Autodesk Inventor part; units mm, degrees
ref_plane "YZ Plane" through (0, 0, 0) normal (1, 0, 0) x (0, 1, 0)
ref_plane "XZ Plane" through (0, 0, 0) normal (0, 1, 0) x (-1, 0, 0)
ref_plane "XY Plane" through (0, 0, 0) normal (0, 0, 1) x (1, 0, 0)
sketch "Szkic1" plane through (0, 0, 0) normal (0, 0, 1) x (1, 0, 0)
  circle A0 centre (0, 0) radius 32.5
  dimension "d0" = 65
extrude "Wyciągnięcie proste1" add sketch "Szkic1" along normal blind 110
ref_plane "Płaszczyzna konstrukcyjna5" through (0, 0, 55) normal (0, 0, -1) x (-1, 0, 0)
sketch "Szkic3" plane through (0, 0, 55) normal (0, 0, -1) x (-1, 0, 0)
  line L0 (0, 0) -> (28, 0)
  line L1 (28, 0) -> (28, 16.5)
  circle A0 centre (0, 0) radius 32.5
  line L2 (28, 0) -> (28, -35.6443)
  line L3 (28, -35.6443) -> (-28, -35.6443)
  line L4 (-28, -35.6443) -> (-28, 35.8328)
  line L5 (-28, 35.8328) -> (28, 35.8328)
  line L6 (28, 35.8328) -> (28, 0)
  dimension "d3" = 28
  dimension "d4" = 56
  dimension "d5" = 56
extrude "Wyciągnięcie proste2" cut sketch "Szkic3" along normal blind 25 and the other way blind 52 contours L2 A0 L4 L1 | A0 L4 L5 L6 | L2 L3 L4 A0
sketch "Szkic5" plane through (0, 0, 0) normal (0, 0, -1) x (-1, 0, 0)
  circle A0 centre (0, 0) radius 32.5
extrude "Wyciągnięcie proste3" cut sketch "Szkic5" against normal blind 27
sketch "Szkic6" plane through (0, 0, 27) normal (0, 0, -1) x (-1, 0, 0)
  circle A0 centre (0, 0) radius 15
  circle A1 centre (0, 0) radius 16.5
  dimension "d12" = 30
  dimension "d13" = 33
extrude "Wyciągnięcie proste4" add sketch "Szkic6" along normal blind 15
sketch "Szkic7" plane through (0, 0, 27) normal (0, 0, -1) x (-1, 0, 0)
  line L0 (7, -15.9899) -> (-7, -15.9899)
  line L1 (-7, -15.9899) -> (-7, -29.9899)
  line L2 (-7, -29.9899) -> (7, -29.9899)
  line L3 (7, -29.9899) -> (7, -15.9899)
  line L4 (7, -15.9899) -> (-7, -29.9899) construction
  line L5 (-7, -15.9899) -> (7, -29.9899) construction
  point P0 (0, 0)
  point P1 (0, -22.9899)
  dimension "d16" = 14
  dimension "d17" = 14
extrude "Wyciągnięcie proste5" cut sketch "Szkic7" along normal blind 5 and the other way blind 7.5
sketch "Szkic8" plane through (28, -16.5, 107) normal (-1, 0, 0) x (0, 0, 1)
  line L0 (-77, 0) -> (-77, 33)
  line L1 (-77, 16.5) -> (-37, 16.5)
  line L2 (0, 0) -> (0, 33)
  line L3 (-37, 16.5) -> (-37, 17.5)
  line L4 (-37, 17.5) -> (-37, 15.5)
  line L5 (-37, 15.5) -> (-77, 15.5)
  line L6 (-77, 15.5) -> (-77, 18.2624)
  line L7 (-77, 15.5) -> (-77, 17.5)
  line L8 (-77, 33) -> (-77, 0)
  line L9 (-77, 17.5) -> (-37, 17.5)
  line L10 (-20, 18.2624) -> (0, 18.2624)
  line L11 (0, 18.2624) -> (0, 16.2624)
  line L12 (0, 16.2624) -> (-20, 16.2624)
  line L13 (-20, 16.2624) -> (-20, 18.2624)
  point P0 (-107, 16.5)
  dimension "d22" = 40
  dimension "d23" = 1
  dimension "d24" = 2
  dimension "d25" = 2
  dimension "d28" = 2
  dimension "d29" = 20
extrude "Wyciągnięcie proste6" add sketch "Szkic8" along normal blind 56
sketch "Szkic9" plane through (0, 0, 110) normal (0, 0, 1) x (1, 0, 0)
  line L0 (12, -27) -> (-12, -27)
  line L1 (-12, -27) -> (-12, -3)
  line L2 (-12, -3) -> (12, -3)
  line L3 (12, -3) -> (12, -27)
  line L4 (12, -27) -> (-12, -3) construction
  line L5 (-12, -27) -> (12, -3) construction
  point P0 (0, 0)
  point P1 (0, -15)
  dimension "d30" = 24
  dimension "d31" = 24
extrude "Wyciągnięcie proste7" cut sketch "Szkic9" against normal blind 56
fillet "Zaokrąglenie1" radius 1 4 edges at (12, -27, 108.5) (-12, -27, 108.5) (12, -3, 108.5) (-12, -3, 108.5)
sketch "Szkic13" plane through (28, -1, 30) normal (0, -1, 0) x (1, 0, 0)
  point P0 (-28, -30)
properties part number "Korpus"
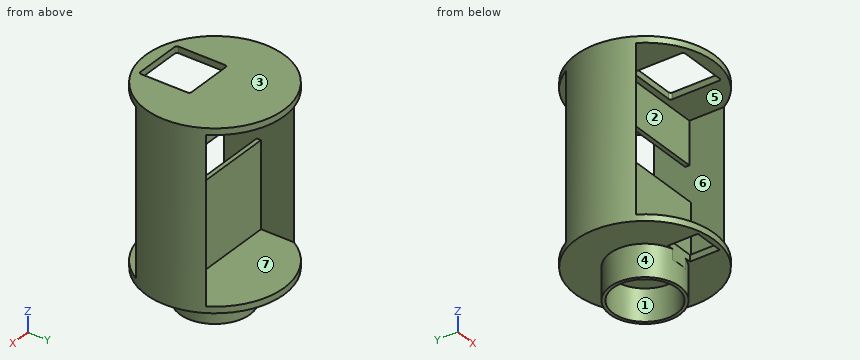
Source: CAD feature listing. Evaluate the final solid. Frame: model axes, mm. Face numbers are marked on the shaded views. A direction names the side the tool comes from. Give positions to 0.01 mm unless a question says otherwise; leave off trailing zeros. Order: outer loops, then holes, each group sorted by start corner. A loop starts at its lowest first (then second) coordinate and runs counter-clockwise, first axis right, second up.
(1) Contact query for flat-ended pins moving along their axis: P1, Ø2.5, axis at x = 0.5, z = 109, coming from the +Y side; P2, Ø12, axis at x = -8, z = 56, coming from the +Y side; P3, Ø1.5, axis at x = 22, y = -0.5, coming from the -Z side; P4, Ø1.5, axis at y = -22.5, z = 28.5, coming from the -X side. Output: stop coordinate, or through.
(2) Access query for the marked faces 5, 6 and 7. Directions: +Z, -Z, +X, -X, +Y, -Y. A direction counts if a zero-diameter tool reaches every point of the face in a straight line with its end or side. Return the directions, or none.
(3) Section query C-C (x = 19.5). Return the cut outline in (y, z).
(4) Section query A-A (x = 0). State how many separate pieces and enclosed holes the cut face has, plus the area to 3 significant figures.
(5) Section query D-D (y = -6.5). Return the cut outline in (x, z), plus the area to 3 significant figures.
(6) Section query B-B (z = 98.5). Return the cut outline in (x, y), plus the area to 3 significant figures.
(7) Pull-direction query (Y, two-part tool) for the marked faces 1, 2, 3 and 4; classes: +Y half, -Y half, draft (parallel to the pull), parting line (faces both ways), or undercut.
(8) Material intervals for line 1 along Z through (x, y) = (12.5, 7.5); line 2 along Y through (x, z) = (0, 24.25); line 3 along Y through (x, z) = (0, 16), sorted ascending.
Outcome:
1. P1: stops at y = 32.5
1. P2: stops at y = 1
1. P3: stops at z = 27
1. P4: stops at x = -24.15
2. face 5: -Y
2. face 6: none
2. face 7: +Y
3. outline: (-26, 27) - (26, 27) - (26, 30) - (1, 30) - (1, 70) - (-1, 70) - (-1, 30) - (-26, 30) - close; (-26, 107) - (-0.24, 107) - (-0.24, 87) - (1.76, 87) - (1.76, 107) - (26, 107) - (26, 110) - (-26, 110) - close
4. separate pieces: 4
4. enclosed holes: 0
4. area: 438 mm2
5. outline: (-31.84, 27) - (-15.17, 27) - (-15.17, 12) - (-13.52, 12) - (-13.52, 27) - (13.52, 27) - (13.52, 12) - (15.17, 12) - (15.17, 27) - (31.84, 27) - (31.84, 110) - (12, 110) - (12, 107) - (28, 107) - (28, 30) - (-28, 30) - (-28, 107) - (-12, 107) - (-12, 110) - (-31.84, 110) - close
5. area: 951 mm2
6. outline: (-28, -16.5) - (-28, -0.24) - (28, -0.24) - (28, -16.5) arc R32.5 ccw to (28, 16.5) - (28, 1.76) - (-28, 1.76) - (-28, 16.5) arc R32.5 ccw to start
6. area: 313 mm2
7. face 1: undercut
7. face 2: -Y half
7. face 3: draft
7. face 4: parting line
8. line 1: z = 27 to 30, 107 to 110
8. line 2: y = -15.99 to -15, 15 to 16.5
8. line 3: y = -16.5 to -15, 15 to 16.5
